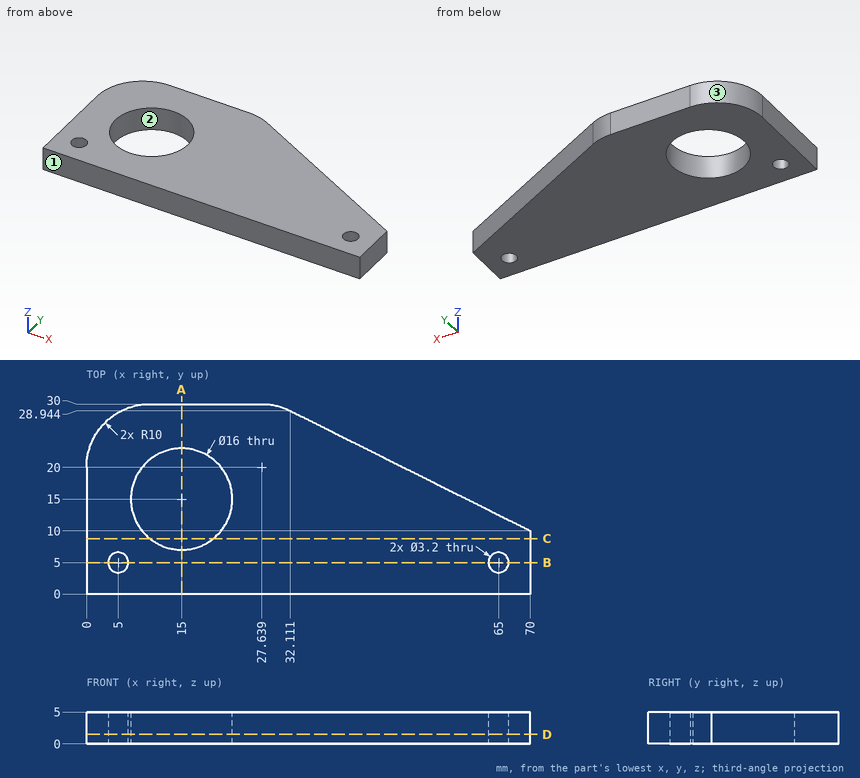
Drawing for the job (mm, zero at the part's lowest x, y, z). Round coordinates to 2 decimals unless told otherwise and drop trailing zeros. Write each loop counter-clockwise with the first axis right and the second up, starting at its lowest first coordinate (ties: lowest second). Pieces come first, ordered by that corner, then holes. Notation, with made-up numbers: (-22, 67) - (-3, 67) arc R11 cw to (-3, 88) - close; hole circle Ø4 at (26.25, 61). An arc over 180 degrees is marked (long way). Write item = value, one per line. Start each with the question number.
Q1. Mould opens along X. For the marked faces 1, 2 and 3 say: pulls with the +X half, pulls with the -X half, needs draft (parallel to the pull), parting line crosses it, or undercut.
Q2. Drop flat-ended pins along their axis: pin 1 (2 mm diameter, centred on y = 26, z = 3.5, fed in from -X); pin 2 (2 mm diameter, centred on y = 21, z = 3, fed in from +X). Give the stop position or say it passes through.
Q3. Band-saw the part on B-B (y = 5). Give the cut face in (x, z), then the cut area to 3 significant figures.
Q4. Band-saw the part on C-C (y = 8.75). Give the cut face in (x, z), then the cut area to 3 significant figures.
Q5. Band-saw the part on D-D (z = 1.5). Give the cut face in (x, y) (1 decimal).
Q6. Band-saw the part on A-A (x = 15). Give the cut face in (y, z), then the cut area to 3 significant figures.
Q7. Probe L1, parallel to X at y = 8.75, z = 3.8 (1 decimal); L2, parallel to X at y = 4.25, z = 4.4 (1 decimal); L3, parallel to X at y = 18.75, z = 3.85 (1 decimal). List the from-to ranges inside material, lowest first. Write a range as from..to.
Answers below:
q1.face_1 = needs draft
q1.face_2 = undercut
q1.face_3 = pulls with the -X half
q2.pin_1 = 1.34
q2.pin_2 = 50
q3.outline = (0, 0) - (3.4, 0) - (3.4, 5) - (0, 5) - close; (6.6, 0) - (63.4, 0) - (63.4, 5) - (6.6, 5) - close; (66.6, 0) - (70, 0) - (70, 5) - (66.6, 5) - close
q3.area = 318 mm2
q4.outline = (0, 0) - (10.01, 0) - (10.01, 5) - (0, 5) - close; (19.99, 0) - (70, 0) - (70, 5) - (19.99, 5) - close
q4.area = 300 mm2
q5.outline = (0, 0) - (70, 0) - (70, 10) - (32.1, 28.9) arc R10 ccw to (27.6, 30) - (10, 30) arc R10 ccw to (0, 20) - close; hole circle Ø3.2 at (5, 5); hole circle Ø16 at (15, 15); hole circle Ø3.2 at (65, 5)
q6.outline = (0, 0) - (7, 0) - (7, 5) - (0, 5) - close; (23, 0) - (30, 0) - (30, 5) - (23, 5) - close
q6.area = 70.0 mm2
q7.L1 = 0..10, 20..70
q7.L2 = 0..3.6, 6.4..63.6, 66.4..70
q7.L3 = 0..7.9, 22.1..52.5
